from build123d import *

# Parameters (mm, degrees)
F1_DEPTH = 50
F2_R     = 10
F3_DEPTH = 65
F4_R     = 10
F5_DEPTH = 35


with BuildPart() as f1:
    # F0 (on Front) → F1 (new body)
    with BuildSketch(Plane.XZ):
        Polygon((20.5, 5), (25.5, 0), (46.5, 0), (51.5, 5), align=None)
        Polygon((25.5, 0), (0, 0), (0, -24.5), (5.5, -19.5), (5.5, -52.5), (0, -47.5), (0, -72), (72, -72), (72, 0), (46.5, 0), align=None)
    extrude(amount=F1_DEPTH)

    # F2 (on face) → F3 (cut)
    with BuildSketch(Plane.YZ.offset(72)):
        with Locations((-25, -20)):
            Circle(F2_R)
    extrude(amount=-F3_DEPTH, mode=Mode.SUBTRACT)

    # F4 (on face) → F5 (cut)
    with BuildSketch(Plane(origin=(0, 0, -72), x_dir=(1, 0, 0), z_dir=(0, 0, -1))):
        with Locations((51, 24.231146)):
            Circle(F4_R)
        with Locations((21.009854, 25)):
            Circle(F4_R)
    extrude(amount=-F5_DEPTH, mode=Mode.SUBTRACT)


solid = f1.part
Geometry: final body of the model. Coordinates: model frame, mm. A direction names the side the tool comes from. Coordinates: 2 decimals unless noted, no trailing zeros. Loops run counter-clockwise (first coordinate to the right, second up) from the corner with the lowest first, then second, coordinate; pieces in that order, holes last. Notation, with made-up numbers: (-21, -7) - (-16, -7) arc R23 ccw to (-16, 7) - close; hole circle Ø2 at (67.5, 78.5). An arc over 180 degrees is marked (long way). One line per question, with ' | ' between items. Start each with the question number.
(1) Cut plane C-C on z = -55.5. Output: boundary loops of the cut face in (x, y), and give its area (3 significant figures).
(2) First-contact query: pin 1 (6 mm diameter, centred on y = -29.5, z = -16.5, fed in from +X); pin 2 (12 mm diameter, centred on x = 15, y = -13.5, fed in from +Z); pin 3 (10 mm diameter, centred on x = 49, y = -28.5, fed in from -Z); pin 4 (8 mm diameter, centred on x = 9.5, y = -19, fed in from +Z). Flat tips, straight axial feed; report the tip coordinate or a pass-through.
(3) Cut plane B-B on y = -41. Output: boundary loops of the cut face in (x, z), and give its area (3 significant figures).
(4) Draft query along Y for faces 4 (the flat face through (21, -25, -37)), 5 (the flat face through (0, -25, -60)), 6 (the flat face through (35, 0, -33)). Return one class per face: +Y half, -Y half, draft (parallel to the pull), parting line (faces both ways), or undercut.
(5) Cut plane D-D on y = -28.5. Output: boundary loops of the cut face in (x, z), and give its area (3 significant figures).
(6) Cut plane A-A on x = 15.5. Output: boundary loops of the cut face in (y, z).
(7) Ray query, L1, parallel to X at y = -32, z = -60.5; L2, parallel to Y at x = 51, z = -65; L3, parallel to Z at x = 41, y = -25. Return the intervals inside material, ascending. Write a range as from..to.
(8) Reachability of faces 1 (the flat face through (5.5, -25, -36)), 2 (the flat face through (13, -25, 0)), 3 (the cylindrical face through (26.39, -33.43, -54.74)) from +Z, -Z, +X, -X, +Y, -Y: full face, straight path, thin tool, end or side. Return the list, or none.
Here are the results:
1) outline: (0, -50) - (72, -50) - (72, 0) - (0, 0) - close; hole circle Ø20 at (21.01, -25); hole circle Ø20 at (51, -24.23) | area: 2,970 mm²
2) pin 1: x = 7 | pin 2: z = 5 | pin 3: z = -37 | pin 4: z = 0
3) outline: (0, -72) - (72, -72) - (72, 0) - (46.5, 0) - (51.5, 5) - (20.5, 5) - (25.5, 0) - (0, 0) - (0, -24.5) - (5.5, -19.5) - (5.5, -52.5) - (0, -47.5) - close | area: 5,160 mm²
4) face 4: undercut | face 5: draft | face 6: +Y half
5) outline: (0, -72) - (11.64, -72) - (11.64, -37) - (30.38, -37) - (30.38, -72) - (41.96, -72) - (41.96, -37) - (60.04, -37) - (60.04, -72) - (72, -72) - (72, -29.37) - (7, -29.37) - (7, -10.63) - (72, -10.63) - (72, 0) - (46.5, 0) - (51.5, 5) - (20.5, 5) - (25.5, 0) - (0, 0) - (0, -24.5) - (5.5, -19.5) - (5.5, -52.5) - (0, -47.5) - close | area: 2,650 mm²
6) outline: (-50, -72) - (-33.35, -72) - (-33.35, -37) - (-16.65, -37) - (-16.65, -72) - (0, -72) - (0, 0) - (-50, 0) - close; hole circle Ø20 at (-25, -20)
7) L1: 0..13.87, 28.15..44.7, 57.3..72 | L2: -50..-34.23, -14.23..0 | L3: -72..-30, -10..5
8) face 1: +Y, -Y | face 2: -X, +Y, -Y | face 3: -Z
